Geometry check sheet. Reference: the model listing, model coordinates, mm. Face numbers are marked on the shaded views. Give positions to 0.01 mm unless a question says otherwise; leave off trailing zeros. Loops run counter-clockwise (first coordinate to the right, second up) from the corner with the lowest first, then second, coordinate; pieces in that order, holes last. Notation, with made-up numbers: (41.25, 47) - (85.25, 47) arc R17 cw to (85.25, 67) - close; hole circle Ø5 at (-37.75, -38). An arc over 180 degrees is marked (long way). Use a Markdown table: item, result. Add a question column.
1. Cross-section at A-A on x = -10.5. Enter the section's corners in (y, z), and give its area (3 significant figures).
2. Cross-section at D-D on x = 10.5. Enter the section's corners in (y, z), and give its area (3 significant figures).
3. Cross-section at B-B on y = -27.5. Enter the section's corners in (x, z).
4. Draft check along Y on the marked faces 1, 2, 3 and 4. Enter one of: pulls with the +Y half, pulls with the -Y half, needs draft (parallel to the pull), parting line crosses it, or undercut.
5. Cross-section at C-C on x = 30.5. Enter the section's corners in (y, z), and give its area (4 significant figures).
6. Material ranges on L1, parallel to X at y = -33.5, z = 0.25; L2, parallel to Y at x = 8, z = 2; L3, parallel to Y at x = 27, z = 2.1, recorded low to high.
from build123d import *

# Parameters (mm, degrees)
F1_DEPTH      = 3
F1_DEPTH_BACK = 3
F2_W          = 105.405718
F2_H          = 2
F3_DEPTH      = 6


with BuildPart() as f1:
    # F0 (on Top) → F1 (new body, two sides)
    with BuildSketch(Plane.XY) as f1_sk:
        with BuildLine():
            ThreePointArc((-2.75, 0), (-2.525174, 1.089034), (-1.887459, 2))
            Line((-1.887459, 2), (-3.172144, 2))
            ThreePointArc((-3.172144, 2), (-3.602641, 1.040903), (-3.75, 0))
            Line((-3.75, 0), (-2.75, 0))
        make_face()
        with BuildLine():
            ThreePointArc((0, -2.75), (-1.944544, -1.944544), (-2.75, 0))
            Line((-2.75, 0), (-3.75, 0))
            ThreePointArc((-3.75, 0), (-2.65165, -2.65165), (0, -3.75))
            Line((0, -3.75), (0, -2.75))
        make_face()
        with BuildLine():
            ThreePointArc((-3.75, 0), (-3.602641, 1.040903), (-3.172144, 2))
            Line((-3.172144, 2), (-6.75, 2))
            ThreePointArc((-6.75, 2), (-6.376894, 1.030776), (-6.25, 0))
            Line((-6.25, 0), (-3.75, 0))
        make_face()
        with BuildLine():
            ThreePointArc((2.75, 0), (1.944544, -1.944544), (0, -2.75))
            Line((0, -2.75), (0, -3.75))
            ThreePointArc((0, -3.75), (2.65165, -2.65165), (3.75, 0))
            Line((3.75, 0), (2.75, 0))
        make_face()
        with BuildLine():
            ThreePointArc((0, -3.75), (-2.65165, -2.65165), (-3.75, 0))
            Line((-3.75, 0), (-6.25, 0))
            Line((-6.25, 0), (-7.25, 0))
            ThreePointArc((-7.25, 0), (-10.5, -3.25), (-13.75, 0))
            Line((-13.75, 0), (-14.75, 0))
            Line((-14.75, 0), (-16.75, 0))
            Line((-16.75, 0), (-17.25, 0))
            Line((-17.25, 0), (-17.75, 0))
            ThreePointArc((-17.75, 0), (-22.057557, -3.073121), (-23.561738, 2))
            Line((-23.561738, 2), (-24.172144, 2))
            Line((-24.172144, 2), (-24.75, 2))
            ThreePointArc((-24.75, 2), (-25.123106, 1.030776), (-25.25, 0))
            Line((-25.25, 0), (-27.75, 0))
            Line((-27.75, 0), (-28.25, 0))
            ThreePointArc((-28.25, 0), (-31.5, -3.25), (-34.75, 0))
            Line((-34.75, 0), (-38, 0))
            Line((-38, 0), (-38, -45))
            Line((-38, -45), (0, -45))
            Line((0, -45), (0, -35))
            Line((0, -35), (-28, -35))
            Line((-28, -35), (-28, -10))
            Line((-28, -10), (0, -10))
            Line((0, -10), (0, -3.75))
        make_face()
        with BuildLine():
            ThreePointArc((-6.25, 0), (-6.376894, 1.030776), (-6.75, 2))
            Line((-6.75, 2), (-7.327856, 2))
            Line((-7.327856, 2), (-7.938262, 2))
            ThreePointArc((-7.938262, 2), (-7.426879, 1.057557), (-7.25, 0))
            Line((-7.25, 0), (-6.25, 0))
        make_face()
        with BuildLine():
            ThreePointArc((1.887459, 2), (2.525174, 1.089034), (2.75, 0))
            Line((2.75, 0), (3.75, 0))
            ThreePointArc((3.75, 0), (3.602641, 1.040903), (3.172144, 2))
            Line((3.172144, 2), (1.887459, 2))
        make_face()
        with BuildLine():
            ThreePointArc((3.75, 0), (2.65165, -2.65165), (0, -3.75))
            Line((0, -3.75), (0, -10))
            Line((0, -10), (28, -10))
            Line((28, -10), (28, -35))
            Line((28, -35), (0, -35))
            Line((0, -35), (0, -45))
            Line((0, -45), (38, -45))
            Line((38, -45), (38, 0))
            Line((38, 0), (34.25, 0))
            Line((34.25, 0), (33.25, 0))
            ThreePointArc((33.25, 0), (30.5, -2.75), (27.75, 0))
            Line((27.75, 0), (26.75, 0))
            ThreePointArc((26.75, 0), (26.897359, 1.040903), (27.327856, 2))
            Line((27.327856, 2), (24.172144, 2))
            Line((24.172144, 2), (22.887459, 2))
            ThreePointArc((22.887459, 2), (22.089034, -2.525174), (18.25, 0))
            Line((18.25, 0), (17.25, 0))
            Line((17.25, 0), (14.25, 0))
            Line((14.25, 0), (13.25, 0))
            ThreePointArc((13.25, 0), (10.5, -2.75), (7.75, 0))
            Line((7.75, 0), (6.75, 0))
            Line((6.75, 0), (3.75, 0))
        make_face()
        with BuildLine():
            ThreePointArc((3.172144, 2), (3.602641, 1.040903), (3.75, 0))
            Line((3.75, 0), (6.75, 0))
            ThreePointArc((6.75, 0), (6.897359, 1.040903), (7.327856, 2))
            Line((7.327856, 2), (3.172144, 2))
        make_face()
        with BuildLine():
            ThreePointArc((7.327856, 2), (6.897359, 1.040903), (6.75, 0))
            Line((6.75, 0), (7.75, 0))
            ThreePointArc((7.75, 0), (7.974826, 1.089034), (8.612541, 2))
            Line((8.612541, 2), (7.327856, 2))
        make_face()
        with BuildLine():
            Line((-14.75, 0), (-13.75, 0))
            ThreePointArc((-13.75, 0), (-13.573121, 1.057557), (-13.061738, 2))
            Line((-13.061738, 2), (-13.672144, 2))
            Line((-13.672144, 2), (-14.25, 2))
            ThreePointArc((-14.25, 2), (-14.623106, 1.030776), (-14.75, 0))
        make_face()
        with BuildLine():
            Line((-16.75, 0), (-14.75, 0))
            ThreePointArc((-14.75, 0), (-14.623106, 1.030776), (-14.25, 2))
            Line((-14.25, 2), (-17.25, 2))
            ThreePointArc((-17.25, 2), (-16.876894, 1.030776), (-16.75, 0))
        make_face()
        with BuildLine():
            ThreePointArc((12.387459, 2), (13.025174, 1.089034), (13.25, 0))
            Line((13.25, 0), (14.25, 0))
            ThreePointArc((14.25, 0), (14.102641, 1.040903), (13.672144, 2))
            Line((13.672144, 2), (12.387459, 2))
        make_face()
        with BuildLine():
            Line((-17.25, 0), (-16.75, 0))
            ThreePointArc((-16.75, 0), (-16.876894, 1.030776), (-17.25, 2))
            Line((-17.25, 2), (-17.827856, 2))
            Line((-17.827856, 2), (-18.438262, 2))
            ThreePointArc((-18.438262, 2), (-17.926879, 1.057557), (-17.75, 0))
            Line((-17.75, 0), (-17.25, 0))
        make_face()
        with BuildLine():
            ThreePointArc((13.672144, 2), (14.102641, 1.040903), (14.25, 0))
            Line((14.25, 0), (17.25, 0))
            ThreePointArc((17.25, 0), (17.397359, 1.040903), (17.827856, 2))
            Line((17.827856, 2), (13.672144, 2))
        make_face()
        with BuildLine():
            Line((-38, 2), (-38, 0))
            Line((-38, 0), (-34.75, 0))
            ThreePointArc((-34.75, 0), (-34.573121, 1.057557), (-34.061738, 2))
            Line((-34.061738, 2), (-38, 2))
        make_face()
        with BuildLine():
            Line((34.25, 0), (38, 0))
            Line((38, 0), (38, 2))
            Line((38, 2), (33.672144, 2))
            ThreePointArc((33.672144, 2), (34.102641, 1.040903), (34.25, 0))
        make_face()
        with BuildLine():
            ThreePointArc((17.827856, 2), (17.397359, 1.040903), (17.25, 0))
            Line((17.25, 0), (18.25, 0))
            ThreePointArc((18.25, 0), (18.474826, 1.089034), (19.112541, 2))
            Line((19.112541, 2), (17.827856, 2))
        make_face()
        with BuildLine():
            Line((33.25, 0), (34.25, 0))
            ThreePointArc((34.25, 0), (34.102641, 1.040903), (33.672144, 2))
            Line((33.672144, 2), (32.387459, 2))
            ThreePointArc((32.387459, 2), (33.025174, 1.089034), (33.25, 0))
        make_face()
        with BuildLine():
            ThreePointArc((-28.938262, 2), (-28.426879, 1.057557), (-28.25, 0))
            Line((-28.25, 0), (-27.75, 0))
            Line((-27.75, 0), (-25.25, 0))
            ThreePointArc((-25.25, 0), (-25.123106, 1.030776), (-24.75, 2))
            Line((-24.75, 2), (-27.327856, 2))
            Line((-27.327856, 2), (-28.612541, 2))
            Line((-28.612541, 2), (-28.938262, 2))
        make_face()
        with BuildLine():
            Line((26.75, 0), (27.75, 0))
            ThreePointArc((27.75, 0), (27.974826, 1.089034), (28.612541, 2))
            Line((28.612541, 2), (27.327856, 2))
            ThreePointArc((27.327856, 2), (26.897359, 1.040903), (26.75, 0))
        make_face()
    extrude(amount=F1_DEPTH)
    extrude(f1_sk.sketch, amount=-F1_DEPTH_BACK)

    # F2 (on face) → F3 (cut)
    with BuildSketch(Plane.XZ.offset(45)):
        Rectangle(F2_W, F2_H)
    extrude(amount=-F3_DEPTH, mode=Mode.SUBTRACT)


solid = f1.part
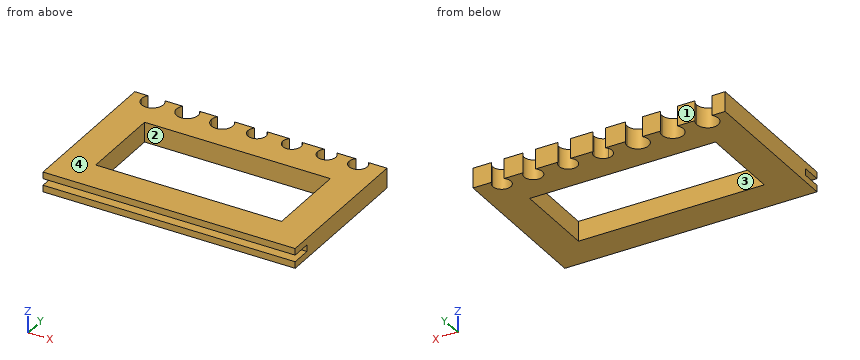
Values found:
| question | item | result |
|---|---|---|
| 1 | outline | (-45, -3) - (-35, -3) - (-35, 3) - (-45, 3) - (-45, 1) - (-39, 1) - (-39, -1) - (-45, -1) - close; (-10, -3) - (-3.25, -3) - (-3.25, 3) - (-10, 3) - close |
| 1 | area | 88.5 mm2 |
| 2 | outline | (-45, -3) - (-35, -3) - (-35, 3) - (-45, 3) - (-45, 1) - (-39, 1) - (-39, -1) - (-45, -1) - close; (-10, -3) - (-2.75, -3) - (-2.75, 3) - (-10, 3) - close |
| 2 | area | 91.5 mm2 |
| 3 | outline | (-38, -3) - (-28, -3) - (-28, 3) - (-38, 3) - close; (28, -3) - (38, -3) - (38, 3) - (28, 3) - close |
| 4 | face 1 | pulls with the +Y half |
| 4 | face 2 | undercut |
| 4 | face 3 | undercut |
| 4 | face 4 | needs draft |
| 5 | outline | (-45, -3) - (-2.75, -3) - (-2.75, 3) - (-45, 3) - (-45, 1) - (-39, 1) - (-39, -1) - (-45, -1) - close |
| 5 | area | 241.5 mm2 |
| 6 | L1 | x = -38 to -28, 28 to 38 |
| 6 | L2 | y = -45 to -35, -10 to -1.15, 1.15 to 2 |
| 6 | L3 | y = -45 to -35, -10 to 2 |
